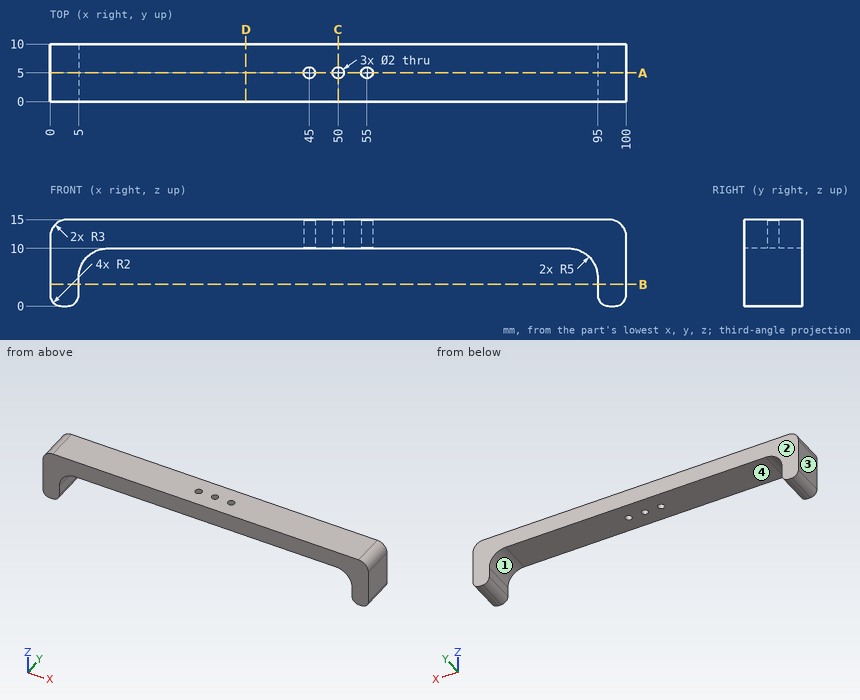
Drawing for the job (mm, zero at the part's lowest x, y, z). Give positions to 0.01 mm unless a question says otherwise; leave off trailing zeros. Loops run counter-clockwise (first coordinate to the right, second up) from the corner with the lowest first, then second, coordinate; pieces in that order, holes last. Notation, with made-up numbers: (-6.75, 76) - (35.25, 76) arc R25 cw to (35.25, 98) - close; hole circle Ø3 at (6, 79). An arc over 180 degrees is marked (long way). Write item = value, one per line. Start each with the question number.
1) Band-saw the part on D-D on x = 34. Give the cut face in (y, z).
2) Band-saw the part on A-A on y = 5. Give the cut face in (x, z), plus the area to 3 significant figures.
3) Band-saw the part on B-B on z = 3.75. Give the cut face in (x, y), plus the area to 3 significant figures.
4) Probe probe 1 along Y at (x, z) = (45, 11.9); probe 2 along Z at (x, y) = (20.5, 8.5); probe 3 along X at (y, z) = (7.5, 4.25). List the from-to ranges inside material, lowest first. Write a range as from..to.
5) Pull direction X, two halves, no side cores. Call the marked faces 1, 2, 3 and 4: +X half, -X half, draft (parallel to the pull), parting line (faces both ways), or undercut.
6) Drop flat-ended pins along their axis: pin 1 Ø1.6 at (x, y) = (45, 5) entering from -Z; pin 2 Ø3 at (x, y) = (55.5, 2) entering from -Z. Give the stop position or say it passes through.
7) Band-saw the part on C-C on x = 50. Give the cut face in (y, z), plus the area to 3 significant figures.
Final values:
q1.outline = (0, 10) - (10, 10) - (10, 15) - (0, 15) - close
q2.outline = (0, 2) arc R2 ccw to (2, 0) - (3, 0) arc R2 ccw to (5, 2) - (5, 5) arc R5 cw to (10, 10) - (44, 10) - (44, 15) - (3, 15) arc R3 ccw to (0, 12) - close; (46, 10) - (49, 10) - (49, 15) - (46, 15) - close; (51, 10) - (54, 10) - (54, 15) - (51, 15) - close; (56, 10) - (90, 10) arc R5 cw to (95, 5) - (95, 2) arc R2 ccw to (97, 0) - (98, 0) arc R2 ccw to (100, 2) - (100, 12) arc R3 ccw to (97, 15) - (56, 15) - close
q2.area = 573 mm²
q3.outline = (0, 0) - (5, 0) - (5, 10) - (0, 10) - close; (95, 0) - (100, 0) - (100, 10) - (95, 10) - close
q3.area = 100 mm²
q4.probe_1 = 0..4, 6..10
q4.probe_2 = 10..15
q4.probe_3 = 0..5, 95..100
q5.face_1 = undercut
q5.face_2 = draft
q5.face_3 = -X half
q5.face_4 = undercut
q6.pin_1 = through
q6.pin_2 = 10
q7.outline = (0, 10) - (4, 10) - (4, 15) - (0, 15) - close; (6, 10) - (10, 10) - (10, 15) - (6, 15) - close
q7.area = 40.0 mm²
